from build123d import *

# Parameters (mm, degrees)
F1_DEPTH = 50.8
F3_DEPTH = 12.701
F5_DEPTH = 12.701


with BuildPart() as f1:
    # F0 (on Right) → F1 (new body)
    with BuildSketch(Plane.YZ):
        Polygon((-24.720795, 16.082145), (-24.720795, 47.832145), (-37.420795, 47.832145), (-37.420795, 28.782145), (-52.681845, 28.782145), (-52.681845, 16.082145), align=None)
    extrude(amount=F1_DEPTH)

    # F2 (on face) → F3 (cut, through all)
    with BuildSketch(Plane.XZ.offset(37.420795)):
        Polygon((31.75, 47.832145), (50.8, 28.782145), (50.8, 47.832145), align=None)
    extrude(amount=-F3_DEPTH, mode=Mode.SUBTRACT)

    # F4 (on face) → F5 (cut, through all)
    with BuildSketch(Plane.XY.offset(28.782145)):
        Polygon((50.8, -52.681845), (50.8, -37.420795), (31.75, -52.681845), align=None)
    extrude(amount=-F5_DEPTH, mode=Mode.SUBTRACT)


solid = f1.part
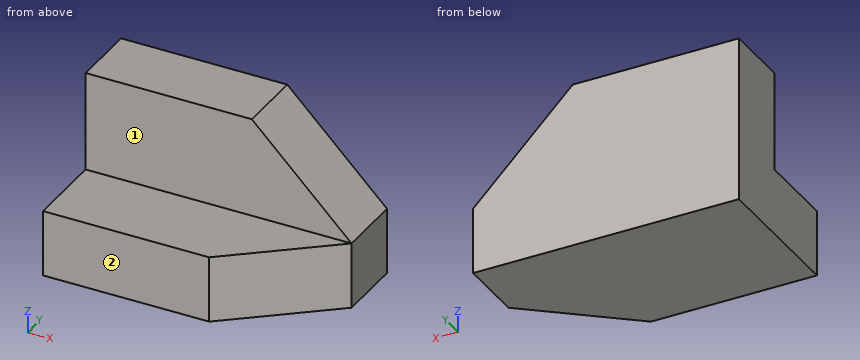
Build history of the part. All positions in model axes, mm. Face numbers are marked on the shaded views. A direction names the side the tool comes from. Round coordinates to 2 decimals unless told otherwise and drop trailing zeros. Write each loop counter-clockwise with the first axis right and the second up, starting at its lowest first coordinate (ties: lowest second). Pieces come first, ordered by that corner, then holes. Notation, with made-up numbers: M 46,64 L 59,64 A18 ccw 59,93 Z; hole C 21.5,69.5 d11. An arc over 180 degrees is marked long. Answer as a JSON object with one key per item and string values. Group by question number.
(1) Cut at C-C (y = -29.75). Give the cut face in (x, z).
(2) Cut at B-B (x = 22). Give the cut face in (y, z).
(3) Which spindle directions (+Z, -Z, +X, -X, +Y, -Y) get a long thin tool onto all of the face, cutting with end or side? Do the marked faces 1 and 2. Say none if no direction does.
(4) Cut at A-A (z = 22). Give the cut face in (x, y), and give its area (3 significant figures).
(5) Flat gauge pins, fed straight in: pin 1 (15 mm diameter, centred on x = 29, z = 39.5, fed in from -Y); pin 2 (12 mm diameter, centred on x = 25.5, y = -48, fed in from +Z). Where does each tip first touch, or does it go through?
(6) Cut at D-D (x = 39). Give the cut face in (y, z).
(7) Drill centre lines: L1, parallel to Y at x = 30, z = 46.5; L2, parallel to Z at x = 20, y = -40; L3, parallel to Y at x = 36, z = 20.5. Where is each one in solid material? Low to high.
Responses:
{
 "1": {"outline": "M 0,16.08 L 50.8,16.08 L 50.8,28.78 L 31.75,47.83 L 0,47.83 Z"},
 "2": {"outline": "M -52.68,16.08 L -24.72,16.08 L -24.72,47.83 L -37.42,47.83 L -37.42,28.78 L -52.68,28.78 Z"},
 "3": {"face 1": "+Z, +X, -X, -Y", "face 2": "+Z, -Z, +X, -X, -Y"},
 "4": {"outline": "M 0,-52.68 L 31.75,-52.68 L 50.8,-37.42 L 50.8,-24.72 L 0,-24.72 Z", "area": "1,280 mm2"},
 "5": {"pin 1": "stops at y = -37.42", "pin 2": "stops at z = 28.78"},
 "6": {"outline": "M -46.87,16.08 L -24.72,16.08 L -24.72,40.58 L -37.42,40.58 L -37.42,28.78 L -46.87,28.78 Z"},
 "7": {"L1": "y = -37.42 to -24.72", "L2": "z = 16.08 to 28.78", "L3": "y = -49.28 to -24.72"}
}
